Geometry check sheet. Reference: the model listing, model coordinates, mm. A direction names the side the tool comes from. Round coordinates to 2 decimals unless told otherwise and drop trailing zeros. Loops run counter-clockwise (first coordinate to the right, second up) from the corner with the lowest first, then second, coordinate; pieces in that order, holes last. Notation, with made-up numbers: M 30.25,73 L 51.25,73 A18 ccw 51.25,81 Z; hole C -16.75,-1.5 d2. An arc over 180 degrees is marked long. Answer in a Markdown table with one row per item. Add a question column.
```python
from build123d import *

# Parameters (mm, degrees)
F0_W      = 99.06
F0_H      = 72.9742
F1_DEPTH  = 0.889
F2_W      = 99.06
F2_H      = 72.9742
F2_W_2    = 96.774
F2_H_2    = 66.8274
F3_DEPTH  = 22.225
F4_R      = 2.032
F6_DEPTH  = 25.4
F8_DEPTH  = 25.4
F10_W     = 6.858
F10_H     = 5.334
F11_DEPTH = 72.9752
F12_W     = 6.858
F12_H     = 0.762
F13_DEPTH = 3.175
F15_W     = 6.858
F15_H     = 5.334
F16_DEPTH = 3.0734
F17_W     = 6.858
F17_H     = 0.762
F18_DEPTH = 3.175


with BuildPart() as f1:
    # F0 (on Top) → F1 (new body)
    with BuildSketch(Plane.XY):
        Rectangle(F0_W, F0_H)
    extrude(amount=F1_DEPTH)

    # F2 (on face) → F3 (join)
    with BuildSketch(Plane(origin=(0, 0, 0), x_dir=(1, 0, 0), z_dir=(0, 0, -1))):
        Rectangle(F2_W, F2_H)
        Rectangle(F2_W_2, F2_H_2, mode=Mode.SUBTRACT)
    extrude(amount=F3_DEPTH)

    # F4
    f4_edges = [f1.edges().sort_by_distance(p)[0] for p in [
        (0, -36.4871, 0.889),
        (49.53, 0, 0.889),
        (0, 36.4871, 0.889),
        (-49.53, 0, 0.889),
    ]]
    fillet(f4_edges, radius=F4_R)

    # F5 (on face) → F6 (cut)
    with BuildSketch(Plane.XY.offset(0.889)):
        Polygon((24.638, -32.0421), (12.446, -32.0421), (12.446, -36.4871), (12.7, -36.4871), (12.7, -32.2961), (24.638, -32.2961), align=None)
        Polygon((38.1, -36.4871), (38.1, -32.0421), (25.908, -32.0421), (25.908, -32.2961), (37.846, -32.2961), (37.846, -36.4871), align=None)
    extrude(amount=-F6_DEPTH, mode=Mode.SUBTRACT)

    # F7 (on face) → F8 (cut)
    with BuildSketch(Plane.XY.offset(0.889)):
        Polygon((12.446, -32.0421), (4.0005, -32.0421), (4.0005, -32.2961), (12.192, -32.2961), (12.192, -36.4871), (12.446, -36.4871), align=None)
        Polygon((2.7305, -32.2961), (2.7305, -32.0421), (-5.715, -32.0421), (-5.715, -36.4871), (-5.461, -36.4871), (-5.461, -32.2961), align=None)
    extrude(amount=-F8_DEPTH, mode=Mode.SUBTRACT)

    # F10 (on face) → F11 (cut, through all)
    with BuildSketch(Plane.XZ.offset(36.4871)):
        with Locations((-25.4, -16.383)):
            Rectangle(F10_W, F10_H)
    extrude(amount=-F11_DEPTH, mode=Mode.SUBTRACT)

    # F12 (on face) → F13 (cut, through all)
    with BuildSketch(Plane(origin=(0, 0, -22.225), x_dir=(1, 0, 0), z_dir=(0, 0, -1))):
        with Locations((-25.4, 33.7947)):
            Rectangle(F12_W, F12_H)
        with Locations((-25.4, -33.7947)):
            Rectangle(F12_W, F12_H)
    extrude(amount=-F13_DEPTH, mode=Mode.SUBTRACT)

    # F15 (on face) → F16 (cut, through all)
    with BuildSketch(Plane(origin=(0, 36.4871, 0), x_dir=(-1, 0, 0), z_dir=(0, 1, 0))):
        with Locations((-25.4, -16.383)):
            Rectangle(F15_W, F15_H)
    extrude(amount=-F16_DEPTH, mode=Mode.SUBTRACT)

    # F17 (on face) → F18 (cut, through all)
    with BuildSketch(Plane(origin=(0, 0, -22.225), x_dir=(1, 0, 0), z_dir=(0, 0, -1))):
        with Locations((25.4, -33.7947)):
            Rectangle(F17_W, F17_H)
    extrude(amount=-F18_DEPTH, mode=Mode.SUBTRACT)


solid = f1.part
```
1) Cross-section at A-A, the plane z = -4.5. Record the boundary of the cut face in (x, y) (3 decimals), plus the area to 3 significant figures.
2) Cross-section at B-B, the plane z = -16. Count the separate pieces of the cut face and the enclosed holes in it, plus the area to 3 significant figures.
3) Set-up check for faces 5 (the flat face through (48.387, 0, -11)), 6 (the flat face through (-49.53, 1, -12)), 7 (the flat face through (12.7, -35, -11)): record each of +Z, -Z, +X, -X, +Y, -Y from which the full face is reachable in a straight line by a thin tool's end or side.
4) Thickness scan on L1, parallel to X at y = -32, z = -17; L2, parallel to Y at x = 37.5, z = -13.75; L3, parallel to Z at x = -10, y = -16. Record the ranges inside material, lowest first. Write a range as [from, to].
5) Cross-section at D-D, the plane x = -39. Record the boundary of the cut face in (y, z) (3 decimals).
6) Cross-section at C-C, the plane y = -9. Record the boundary of the cut face in (x, z) (3 decimals), plus the area to 3 significant figures.
7) Draft check along Z on faces 1 (the cylindrical face through (48.95, 0.51, 0.28)), 2 (the flat face through (25, -33.414, -11)), 3 (the flat face through (25, -35, -22.225)), 4 (the flat face through (-21.971, -35, -17)). Enter one of: +Z half, -Z half, draft (parallel to the pull), parting line (faces both ways), or undercut.
8) Go/stop test with flat-tipped pins: pin 1 (1 mm diameter, centred on x = 33.5, z = 0, fed in from +Y); pin 2 (6 mm diameter, centred on x = 18.5, y = 19, fed in from -Z); pin 3 (0.7 mm diameter, centred on x = -0.5, z = 0.5, fed in from -Y). Record where each tip stops, or that it passes through.
Worked answers:
| question | item | result |
|---|---|---|
| 1 | outline | M -49.53,-36.487 L -5.715,-36.487 L -5.715,-33.414 L -48.387,-33.414 L -48.387,33.414 L 48.387,33.414 L 48.387,-33.414 L 38.1,-33.414 L 38.1,-36.487 L 49.53,-36.487 L 49.53,36.487 L -49.53,36.487 Z; M -5.461,-36.487 L 12.192,-36.487 L 12.192,-33.414 L -5.461,-33.414 Z; M 12.7,-36.487 L 37.846,-36.487 L 37.846,-33.414 L 12.7,-33.414 Z |
| 1 | area | 759 mm2 |
| 2 | separate pieces | 6 |
| 2 | enclosed holes | 0 |
| 2 | area | 695 mm2 |
| 3 | face 5 | -Z |
| 3 | face 6 | +Z, -Z, -X, +Y, -Y |
| 3 | face 7 | +Z, -Z, -Y |
| 4 | L1 | x = [-49.53, -48.39], [48.39, 49.53] |
| 4 | L2 | y = [-36.49, -33.41], [33.41, 36.49] |
| 4 | L3 | z = [0, 0.89] |
| 5 | outline | M -36.487,-22.225 L -33.414,-22.225 L -33.414,0 L 33.414,0 L 33.414,-22.225 L 36.487,-22.225 L 36.487,-1.143 A2.032 ccw 34.455,0.889 L -34.455,0.889 A2.032 ccw -36.487,-1.143 Z |
| 6 | outline | M -49.53,-22.225 L -48.387,-22.225 L -48.387,0 L 48.387,0 L 48.387,-22.225 L 49.53,-22.225 L 49.53,-1.143 A2.032 ccw 47.498,0.889 L -47.498,0.889 A2.032 ccw -49.53,-1.143 Z |
| 6 | area | 137 mm2 |
| 7 | face 1 | +Z half |
| 7 | face 2 | draft |
| 7 | face 3 | -Z half |
| 7 | face 4 | undercut |
| 8 | pin 1 | stops at y = 36.38 |
| 8 | pin 2 | stops at z = 0 |
| 8 | pin 3 | stops at y = -36.02 |
